Job drawing, mm, ordinate dimensions from the low corner. One solid piece. Give positions to 0.01 mm unless a question says otherwise; leave off trailing zeros. Order: outer loops, then holes, each group sorted by start corner. A loop starts at its lowest first (then second) coordinate and runs counter-clockwise, first axis right, second up.
Item 1: Flat gauge pins, fed straight in: P1, Ø2, axis at y = 57, z = 1, coming from the +X side; P2, Ø2, axis at y = 50, z = 1.5, coming from the -X side; P3, Ø1.2, axis at x = 86.5, z = 2.5, coming from the +Y side. Where does each tip first touch, or does it go through?
Item 2: Band-saw the part on B-B on x = 87.5. Give the cut face in (y, z).
Item 3: Band-saw the part on C-C on y = 52. Give the cut face in (x, z), plus the area to 3 significant figures.
Item 4: Wall check: L1, parallel to Y at x = 63, z = 1.95; L2, parallel to X at y = 37.5, z = 2.5; L3, parallel to Y at x = 46.5, z = 1.6 (1 decimal). Give the ranges that are in metal, low to high.
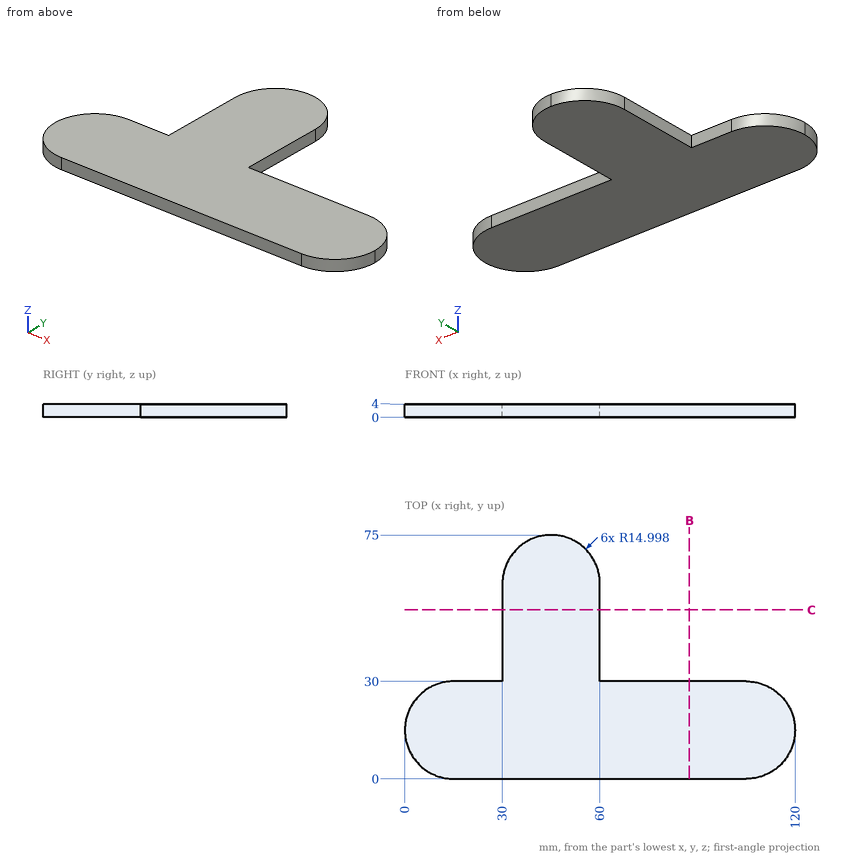
The answers:
1. P1: stops at x = 60
1. P2: stops at x = 30
1. P3: stops at y = 30
2. outline: (0, 0) - (30, 0) - (30, 4) - (0, 4) - close
3. outline: (30, 0) - (60, 0) - (60, 4) - (30, 4) - close
3. area: 120 mm2
4. L1: y = 0 to 30
4. L2: x = 30 to 60
4. L3: y = 0 to 74.9
